For this review, take the finished solid that the model builds, in its own axes (mm). A direction names the side the tool comes from. Give positions to 0.01 mm unless a question says otherwise; leave off trailing zeros. Order: outer loops, then holes, each group sorted by start corner. A loop starts at its lowest first (then second) coordinate and runs counter-clockwise, first axis right, second up. Notation, with made-up numbers: M 55.5,67.5 L 81.5,67.5 A21 cw 81.5,91.5 Z; hole C -17,67 d8. An arc over 180 degrees is marked long. Answer as CSV lines item,"result". Start each with the question number.
1. Machinability: for faces 5 (the flat face through (-3, 4, -3)), 6 (the flat face through (43.28, 12.41, -8.89)), 7 (the cylindrical face through (9.05, 2.96, 0.09)), 8 (the flat face through (86, 6, 0)), which of the approach directions +Z, -Z, +X, -X, +Y, -Y give a long, thin tool a straight path to every point of the face, cutting with its end or side? Answer none if there is none.
2. We need section B-B, the plane x = 44.9. Give the boundary of the cut face in (y, z).
3. Clearance check with flat-ended pins moving along their axes: P1, Ø17, axis at x = 0, z = 0, coming from the +Y side; P2, Ø1.5, axis at y = 3, z = 1, coming from the -X side; P3, Ø1.5, axis at y = 15, z = -3.5, coming from the +X side. State where each tip first meets the part, or that it passes through.
4. For line 1 along Z through (x, y) = (69.5, 4.35); line 2 along X through (y, z) = (15.25, -5.35); line 3 along X through (y, z) = (14.25, 5.25), list the stretches that pass through material, from the lowest coordinate up.
5. We need section A-A, the plane y = 13.75. State how many separate pieces and enclosed holes the cut face has, and give its area (3 significant figures).
6. Mouldability with a two-part tool opening along X and no side actions: class faces 1 (the cylindrical face through (5.523, 1.972, 3.521)), 2 (the flat face through (86.99, 12.41, 1.67)), 3 (the cylindrical face through (-11.5, 3, -0.2)), 4 (the flat face through (87.578, 7.256, -9.437)) as pulls with the +X half, pulls with the -X half, needs draft (parallel to the pull), parting line crosses it, or undercut.
from build123d import *

# Parameters (mm, degrees)
SKETCH1_R           = 1.9
SKETCH1_R_2         = 4.05
SKETCH1_R_3         = 12.3
SKETCH1_R_4         = 1.95
BOSS_EXTRUDE1_DEPTH = 6
SKETCH2_R           = 6.55
CUT_EXTRUDE1_DEPTH  = 4
SKETCH3_R           = 1.9
BOSS_EXTRUDE3_DEPTH = 13
SKETCH4_R           = 1.9
SKETCH4_R_2         = 1.95
BOSS_EXTRUDE4_DEPTH = 13


with BuildPart() as part:
    # Sketch1 → Boss-Extrude1 (new body)
    with BuildSketch(Plane(origin=(0, 0, 0), x_dir=(1, 0, 0), z_dir=(0, 1, 0))):
        with BuildLine():
            Line((68.797266187, 14.783306977), (-0.546043165, 11.48702907))
            ThreePointArc((-0.546043165, 11.48702907), (-11.5, 0), (-0.546043165, -11.48702907))
            Line((-0.546043165, -11.48702907), (68.797266187, -14.783306977))
            ThreePointArc((68.797266187, -14.783306977), (71.590968354, -14.651547746), (74.31, -13.996567436))
            Line((74.31, -13.996567436), (95.775, -6.619998112))
            ThreePointArc((95.775, -6.619998112), (100.5, 0), (95.775, 6.619998112))
            Line((95.775, 6.619998112), (74.31, 13.996567436))
            ThreePointArc((74.31, 13.996567436), (71.590968354, 14.651547746), (68.797266187, 14.783306977))
        make_face()
        with Locations(Location((44.9, -5.35, 0), (0, 0, 270))):
            Circle(SKETCH1_R, mode=Mode.SUBTRACT)
        with Locations(Location((0, 0, 0), (0, 0, 270))):
            Circle(SKETCH1_R_2, mode=Mode.SUBTRACT)
        with BuildLine():
            ThreePointArc((12.898162181, -4.044967428), (9.05, 0), (12.898162181, 4.044967428))
            Line((12.898162181, 4.044967428), (31.975408753, 4.996893474))
            ThreePointArc((31.975408753, 4.996893474), (33.823154358, 4.311281054), (34.6, 2.5))
            Line((34.6, 2.5), (34.6, -2.5))
            ThreePointArc((34.6, -2.5), (33.823154358, -4.311281054), (31.975408753, -4.996893474))
            Line((31.975408753, -4.996893474), (12.898162181, -4.044967428))
        make_face(mode=Mode.SUBTRACT)
        with Locations(Location((44.9, 5.35, 0), (0, 0, 270))):
            Circle(SKETCH1_R, mode=Mode.SUBTRACT)
        with Locations(Location((69.5, 0, 0), (0, 0, 270))):
            Circle(SKETCH1_R_3, mode=Mode.SUBTRACT)
        with Locations(Location((86.96, 5.75, 0), (0, 0, 270))):
            Circle(SKETCH1_R, mode=Mode.SUBTRACT)
        with Locations(Location((95.96, 0, 0), (0, 0, 270))):
            Circle(SKETCH1_R_4, mode=Mode.SUBTRACT)
        with Locations(Location((86.96, -5.75, 0), (0, 0, 270))):
            Circle(SKETCH1_R, mode=Mode.SUBTRACT)
    extrude(amount=BOSS_EXTRUDE1_DEPTH)

    # Sketch2 → Cut-Extrude1 (cut)
    with BuildSketch(Plane(origin=(0, 0, 0), x_dir=(1, 0, 0), z_dir=(0, 1, 0))):
        with Locations(Location((0, 0, 0), (0, 0, 270))):
            Circle(SKETCH2_R)
    extrude(amount=CUT_EXTRUDE1_DEPTH, mode=Mode.SUBTRACT)

    # Sketch3 → Boss-Extrude3 (add)
    with BuildSketch(Plane(origin=(0, 6, 0), x_dir=(1, 0, 0), z_dir=(0, 1, 0))):
        with BuildLine():
            Line((37.810248758, 9.243466249), (48.9, 8.53))
            ThreePointArc((48.9, 8.53), (50.810248758, 0), (48.9, -8.53))
            Line((48.9, -8.53), (37.810248758, -9.243466249))
            ThreePointArc((37.810248758, -9.243466249), (40.074456368, 0), (37.810248758, 9.243466249))
        make_face()
        with Locations(Location((44.9, -5.35, 0), (0, 0, 270))):
            Circle(SKETCH3_R, mode=Mode.SUBTRACT)
        with Locations(Location((44.9, 5.35, 0), (0, 0, 270))):
            Circle(SKETCH3_R, mode=Mode.SUBTRACT)
    extrude(amount=BOSS_EXTRUDE3_DEPTH)

    # Sketch4 → Boss-Extrude4 (add)
    with BuildSketch(Plane(origin=(0, 6, 0), x_dir=(1, 0, 0), z_dir=(0, 1, 0))):
        with BuildLine():
            Line((85.0425, 10.308282774), (79.790912588, 6.736996223))
            ThreePointArc((79.790912588, 6.736996223), (80.683848774, 5.119719388), (81.32449086, 3.386947876))
            Line((81.32449086, 3.386947876), (92.5, 0))
            Line((92.5, 0), (81.32449086, -3.386947876))
            ThreePointArc((81.32449086, -3.386947876), (80.683848774, -5.119719388), (79.790912588, -6.736996223))
            Line((79.790912588, -6.736996223), (85.0425, -10.308282774))
            Line((85.0425, -10.308282774), (95.775, -6.619998112))
            ThreePointArc((95.775, -6.619998112), (100.5, 0), (95.775, 6.619998112))
            Line((95.775, 6.619998112), (85.0425, 10.308282774))
        make_face()
        with Locations(Location((86.96, 5.75, 0), (0, 0, 270))):
            Circle(SKETCH4_R, mode=Mode.SUBTRACT)
        with Locations(Location((86.96, -5.75, 0), (0, 0, 270))):
            Circle(SKETCH4_R, mode=Mode.SUBTRACT)
        with Locations(Location((95.96, 0, 0), (0, 0, 270))):
            Circle(SKETCH4_R_2, mode=Mode.SUBTRACT)
    extrude(amount=BOSS_EXTRUDE4_DEPTH)


solid = part.part
Result set:
1,face 5,"-Y"
1,face 6,"-Z, +Y"
1,face 7,"+Y, -Y"
1,face 8,"+Y"
2,outline,"M 0,-13.65 L 6,-13.65 L 6,-8.79 L 19,-8.79 L 19,-7.25 L 0,-7.25 Z; M 0,-3.45 L 19,-3.45 L 19,3.45 L 0,3.45 Z; M 0,7.25 L 19,7.25 L 19,8.79 L 6,8.79 L 6,13.65 L 0,13.65 Z"
3,P1,"y = 6"
3,P2,"x = -11.5"
3,P3,"x = 99.94"
4,line 1,"-14.8 to -12.3, 12.3 to 14.8"
4,line 2,"39.35 to 43, 46.8 to 50.08, 80.58 to 85.1, 88.82 to 98.01"
4,line 3,"39.37 to 43, 46.8 to 50.11, 80.62 to 85.13, 88.79 to 98.13"
5,separate pieces,"2"
5,enclosed holes,"5"
5,area,"396 mm2"
6,face 1,"undercut"
6,face 2,"undercut"
6,face 3,"pulls with the -X half"
6,face 4,"pulls with the +X half"
